Autodesk Inventor part; units mm, degrees
ref_plane "YZ Plane" through (0, 0, 0) normal (1, 0, 0) x (0, 1, 0)
ref_plane "XZ Plane" through (0, 0, 0) normal (0, 1, 0) x (-1, 0, 0)
ref_plane "XY Plane" through (0, 0, 0) normal (0, 0, 1) x (1, 0, 0)
sketch "Sketch1" plane through (0, 0, 0) normal (1, 0, 0) x (0, 1, 0)
  line L0 (0, 0) -> (19.05, 0)
  line L1 (19.05, 0) -> (19.05, -15.875)
  line L2 (19.05, -15.875) -> (0, -15.875)
  line L3 (0, -15.875) -> (0, 0)
  line L4 (0, 0) -> (15.875, 0)
  line L5 (15.875, 0) -> (15.875, -12.7)
  line L6 (15.875, -12.7) -> (0, -12.7)
  line L7 (0, -12.7) -> (0, 0)
  dimension "d0" = 19.05
  dimension "d1" = 15.875
  dimension "d2" = 15.875
  dimension "d3" = 12.7
extrude "Extrusion1" add sketch "Sketch1" along normal blind 19.05 contours L0 L1 L2 L3 L6 L5
sketch "Sketch2" plane through (0, 19.05, 0) normal (0, 1, 0) x (1, 0, 0)
  line L0 (0, 15.875) -> (0, 0)
  line L1 (0, 0) -> (19.05, 0)
  line L2 (19.05, 15.875) -> (19.05, 0)
  line L3 (0, 15.875) -> (19.05, 15.875)
  point P0 (0, 0)
  point P1 (4.7625, 6.35)
  point P2 (14.2875, 6.35)
  dimension "d6" = 9.525
  dimension "d7" = 4.7625
  dimension "d8" = 15.875
  dimension "d18" = 9.525
  dimension "d19" = 9.525
  dimension "d31" = 19.05
hole "Hole1" at (4.7625, 19.05, -6.35) at (14.2875, 19.05, -6.35) direction (0, -1, 0) diameter 3.429 end through all
sketch "Sketch3" plane through (0, 0, -12.7) normal (0, 0, 1) x (1, 0, 0)
  line L0 (0, 0) -> (0, 15.875)
  line L1 (19.05, 0) -> (0, 0)
  line L2 (19.05, 15.875) -> (19.05, 0)
  line L3 (0, 15.875) -> (19.05, 15.875)
  point P0 (0, 0)
  point P1 (4.7625, 4.7625)
  point P2 (14.2875, 4.7625)
  dimension "d20" = 9.525
  dimension "d21" = 4.7625
  dimension "d22" = 4.7625
  dimension "d23" = 4.7625
  dimension "d32" = 19.05
hole "Hole2" at (4.7625, 4.7625, -12.7) at (14.2875, 4.7625, -12.7) direction (0, 0, -1) diameter 3.81 end through all
properties part number "TensionerPlate3" material "ABS Plastic"
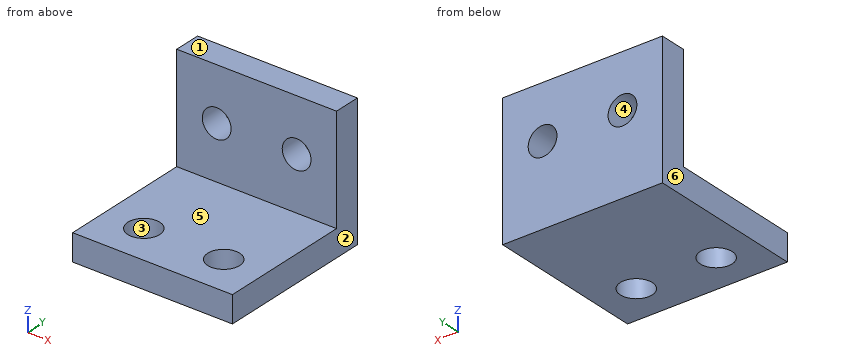
CAD build for the part. Positions are in the model's coordinates, mm. Face numbers are marked on the shaded views. A direction names the side the tool comes from. Round coordinates to 2 decimals unless told otherwise and drop trailing zeros. Order: outer loops, then holes, each group sorted by start corner. A loop starts at its lowest first (then second) coordinate and runs counter-clockwise, first axis right, second up. Notation, with made-up numbers: (-7, -13.5) -> (48, -13.5) arc R23 ccw to (48, 20.5) -> close; hole circle Ø11 at (-22, 19). An arc over 180 degrees is marked (long way). Write item = value, one per line.
(1) Cut at D-D (x = 8). Write the cut outline in (y, z) (3 decimals).
Answers follow:
outline = (0, -15.875) -> (19.05, -15.875) -> (19.05, 0) -> (15.875, 0) -> (15.875, -12.7) -> (0, -12.7) -> close
(2) Pull direction X, two halves, no side cores. Call the marked faces 1, 2, 3 and 4: +X half, -X half, draft (parallel to the pull), parting line (faces both ways), or undercut.
Answers follow:
face_1 = draft
face_2 = +X half
face_3 = undercut
face_4 = undercut
(3) Drill centre lines: L1, parallel to X at y = 17.45, z = -6.35; L2, parallel to Z at x = 16.25, y = 3.5 (3 decimals); L3, parallel to Y at x = 11, z = -7 (3 decimals). Where is each one in solid material? Low to high.
Answers follow:
L1 = 0 to 3.05, 6.48 to 12.57, 16 to 19.05
L2 = -15.875 to -12.7
L3 = 15.875 to 19.05
(4) 3-axis set-ups, long thin cutter, end or side, ignore diameter. For the marked faces 5 and 6: which of +Z, -Z, +X, -X, +Y, -Y reach the whole face in a straight line?
Answers follow:
face_5 = +Z, +X, -X, -Y
face_6 = +Z, -Z, -X, +Y, -Y
(5) Flat gauge pins, fed straight in: P1, Ø8, axis at x = 14, z = -2, coming from the -Y side (3 decimals); P2, Ø8, axis at x = 14.5, y = 11, coming from the +Z side; P3, Ø2.5, axis at x = 4.76, z = -6.35, coming from the +Y side. Where does each tip first touch, or does it go through?
Answers follow:
P1 = 15.875
P2 = -12.7
P3 = through
(6) Cut at A-A (z = -6.35). Write the cut outline in (x, y) (3 decimals), plus the area to 3 significant figures.
Answers follow:
outline = (0, 15.875) -> (3.048, 15.875) -> (3.048, 19.05) -> (0, 19.05) -> close; (6.477, 15.875) -> (12.573, 15.875) -> (12.573, 19.05) -> (6.477, 19.05) -> close; (16.002, 15.875) -> (19.05, 15.875) -> (19.05, 19.05) -> (16.002, 19.05) -> close
area = 38.7 mm²
(7) Cut at B-B (x = 5.75). Write the cut outline in (y, z) (3 decimals).
Answers follow:
outline = (0, -15.875) -> (3.133, -15.875) -> (3.133, -12.7) -> (0, -12.7) -> close; (6.392, -15.875) -> (19.05, -15.875) -> (19.05, -7.752) -> (15.875, -7.752) -> (15.875, -12.7) -> (6.392, -12.7) -> close; (15.875, -4.948) -> (19.05, -4.948) -> (19.05, 0) -> (15.875, 0) -> close
(8) Cut at C-C (y = 4.75). Write the cut outline in (x, z) (3 decimals), plus the area to 3 significant figures.
Answers follow:
outline = (0, -15.875) -> (2.858, -15.875) -> (2.858, -12.7) -> (0, -12.7) -> close; (6.667, -15.875) -> (12.383, -15.875) -> (12.383, -12.7) -> (6.667, -12.7) -> close; (16.192, -15.875) -> (19.05, -15.875) -> (19.05, -12.7) -> (16.192, -12.7) -> close
area = 36.3 mm²
